from build123d import *

# Parameters (mm, degrees)
SKIZZE1_R                       = 3
AUFSATZ_LINEAR_AUSTRAGEN1_DEPTH = 4
SKIZZE3_W                       = 48
SKIZZE3_H                       = 40
SKIZZE3_R                       = 1.324941068
AUFSATZ_LINEAR_AUSTRAGEN2_DEPTH = 4


with BuildPart() as part:
    # Skizze1 → Aufsatz-Linear austragen1 (new body)
    with BuildSketch(Plane.XY):
        Polygon((-78.13229572, 0), (-43.13229572, 0), (-43.13229572, 40), (-25.505836576, 40), (6.86770428, 0), (6.86770428, -40), (-78.13229572, -40), align=None)
        with Locations((-13.13229572, -20)):
            Circle(SKIZZE1_R, mode=Mode.SUBTRACT)
    extrude(amount=AUFSATZ_LINEAR_AUSTRAGEN1_DEPTH)

    # Skizze3 → Aufsatz-Linear austragen2 (add)
    with BuildSketch(Plane.ZY.offset(43.13229572)):
        with Locations((24, 7.085584289)):
            Rectangle(SKIZZE3_W, SKIZZE3_H)
        with Locations((24, 7.085584289)):
            Circle(SKIZZE3_R, mode=Mode.SUBTRACT)
    extrude(amount=-AUFSATZ_LINEAR_AUSTRAGEN2_DEPTH)


solid = part.part
Model file for the job. Use its own axes, mm. A direction names the side the tool comes from. Round coordinates to 2 decimals unless told otherwise and drop trailing zeros. Order: outer loops, then holes, each group sorted by start corner. A loop starts at its lowest first (then second) coordinate and runs counter-clockwise, first axis right, second up.
(1) 3-axis set-ups, long thin cutter, end or side, ignore diameter. For faces 1 (the face through (-61, 0, 2)), 2 (the face through (-41, 27.086, 26)), 3 (the face through (-41, -12.914, 26)): which of +Z, -Z, +X, -X, +Y, -Y reach the whole face in a straight line?
(2) Band-saw the part on D-D (x = -44.5). List the corners of the cut face in (y, z), then the cut area to 3 significant figures.
(3) Band-saw the part on B-B (z = 24). List the corners of the cut face in (x, y).
(4) Pin check, flat tips, straight feed: pin 1 (1 mm diameter, centred on x = -44.5, z = 15, fed in from +Y); pin 2 (3.5 mm diameter, centred on y = 7.09, z = 24, fed in from +X); pin 3 (4.5 mm diameter, centred on x = -41, z = 20, fed in from -Y); pin 4 (4.5 mm diameter, centred on x = -61, z = 1.5, fed in from +Y). Stop position of each tip, or through.
(5) Drill centre lines: line 1 (Y direction, x = -40.5, z = 24); line 2 (Z direction, x = -42, y = 7); line 3 (Z direction, x = -1.5, y = -17). Where is each one in solid material? Low to high.
(6) Pull direction Z, two halves, no side cores. Call faces 4 (the face through (-41.16, 7.484, 25.264)), 5 (the face through (-41, 7, 48)), 6 (the face through (-39.132, 7, 26)): released by +Z, released by -Z, zero draft, split by the parting line, or undercut.
(7) Band-saw the part on C-C (y = -5). List the corners of the cut face in (x, z).
(8) Band-saw the part on A-A (y = -20). List the corners of the cut face in (x, z).
Verdict:
1. face 1: +Z, -Z, -X, +Y
1. face 2: +Z, +X, -X, +Y
1. face 3: +Z, +X, -X, -Y
2. outline: (-40, 0) - (0, 0) - (0, 4) - (-40, 4) - close
2. area: 160 mm2
3. outline: (-43.13, -12.91) - (-39.13, -12.91) - (-39.13, 5.76) - (-43.13, 5.76) - close; (-43.13, 8.41) - (-39.13, 8.41) - (-39.13, 27.09) - (-43.13, 27.09) - close
4. pin 1: passes through
4. pin 2: stops at x = -39.13
4. pin 3: stops at y = -12.91
4. pin 4: stops at y = 0
5. line 1: y = -12.91 to 5.76, 8.41 to 27.09
5. line 2: z = 0 to 22.68, 25.32 to 48
5. line 3: z = 0 to 4
6. face 4: undercut
6. face 5: released by +Z
6. face 6: zero draft
7. outline: (-78.13, 0) - (6.87, 0) - (6.87, 4) - (-39.13, 4) - (-39.13, 48) - (-43.13, 48) - (-43.13, 4) - (-78.13, 4) - close
8. outline: (-78.13, 0) - (-16.13, 0) - (-16.13, 4) - (-78.13, 4) - close; (-10.13, 0) - (6.87, 0) - (6.87, 4) - (-10.13, 4) - close
